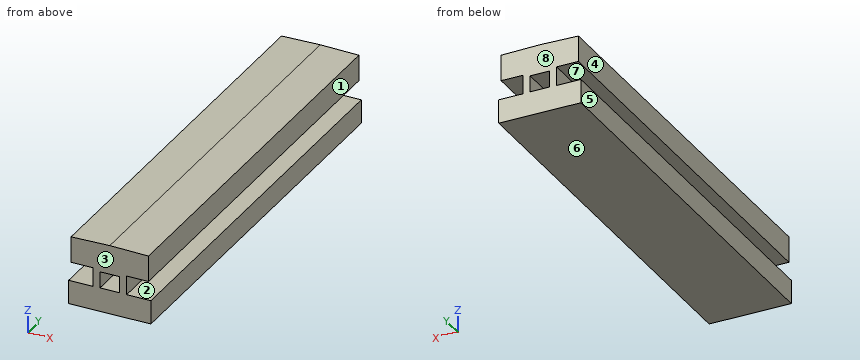
```python
from build123d import *

# Parameters (mm, degrees)
F1_DEPTH = 500
F2_W     = 23.519294
F2_H     = 19.81963
F3_DEPTH = 500


with BuildPart() as f1:
    # F0 (on Front) → F1 (new body)
    with BuildSketch(Plane.XZ):
        Polygon((-49.813338, -38.97861), (0, -38.97861), (49.813338, -38.97861), (49.813338, -10.174078), (20.480286, -10.174078), (20.480286, 12.816695), (46.90646, 12.816695), (46.90646, 44.263847), (0, 45.320891), (-46.90646, 44.263847), (-46.90646, 12.816695), (-20.480286, 12.816695), (-20.480286, -10.174078), (-49.813338, -10.174078), align=None)
    extrude(amount=F1_DEPTH)

    # F2 (on face) → F3 (cut)
    with BuildSketch(Plane.XZ.offset(500)):
        Rectangle(F2_W, F2_H)
    extrude(amount=-F3_DEPTH, mode=Mode.SUBTRACT)


solid = f1.part
```
Geometry check sheet. Reference: the model listing, model coordinates, mm. Face numbers are marked on the shaded views. A direction names the side the tool comes from. Round coordinates to 2 decimals unless told otherwise and drop trailing zeros. Write each loop counter-clockwise with the first axis right and the second up, starting at its lowest first coordinate (ties: lowest second). Pieces come first, ordered by that corner, then holes. Notation, with made-up numbers: (54, 34.25) -> (69, 34.25) arc R21 cw to (69, 58.25) -> close; hole circle Ø7 at (62, 28.25). An arc over 180 degrees is marked (long way). Put each result on its own line as item: value.
1) Thickness scan on probe 1 along X at (y, z) = (-355, 1); probe 2 along Z at (x, y) = (45, -41.5); probe 3 along X at (y, z) = (-142.5, 23). Record the ranges inside material, lowest first. Write a range as from..to.
Recorded:
probe 1: x = -20.48..-11.76, 11.76..20.48
probe 2: z = -38.98..-10.17, 12.82..44.31
probe 3: x = -46.91..46.91
2) Release check for a two-part mould opening along Z. For the marked faces 6, 7 and 8 record: pulls with the +Z half, pulls with the -Z half, needs draft (parallel to the pull), parting line crosses it, or undercut.
Recorded:
face 6: pulls with the -Z half
face 7: undercut
face 8: needs draft
3) Cross-section at A-A, the plane z = -2. Enter the section's corners in (x, y), plus the area to 3 significant figures.
Recorded:
outline: (-20.48, -500) -> (-11.76, -500) -> (-11.76, 0) -> (-20.48, 0) -> close; (11.76, -500) -> (20.48, -500) -> (20.48, 0) -> (11.76, 0) -> close
area: 8,720 mm2
4) Access from +Z, -Z, +X, -X, +Y, -Y to the whole of each face (thin tool, end or side, straight path). Record for the marked faces 1, 2, 3, 4 and 5.
Recorded:
face 1: +Z, +X, +Y, -Y
face 2: +X, +Y, -Y
face 3: +Z, -Z, +X, -X, -Y
face 4: +Z, -X, +Y, -Y
face 5: +Z, -Z, -X, +Y, -Y
5) Cross-section at B-B, the plane y = -334. Enter the section's corners in (x, z).
Recorded:
outline: (-49.81, -38.98) -> (49.81, -38.98) -> (49.81, -10.17) -> (20.48, -10.17) -> (20.48, 12.82) -> (46.91, 12.82) -> (46.91, 44.26) -> (0, 45.32) -> (-46.91, 44.26) -> (-46.91, 12.82) -> (-20.48, 12.82) -> (-20.48, -10.17) -> (-49.81, -10.17) -> close; hole (-11.76, -9.91) -> (11.76, -9.91) -> (11.76, 9.91) -> (-11.76, 9.91) -> close
6) Cross-section at C-C, the plane x = 26. Enter the section's corners in (y, z), plus the area to 3 significant figures.
Recorded:
outline: (-500, -38.98) -> (0, -38.98) -> (0, -10.17) -> (-500, -10.17) -> close; (-500, 12.82) -> (0, 12.82) -> (0, 44.73) -> (-500, 44.73) -> close
area: 30,400 mm2
7) Cross-section at D-D, the plane z = 36. Enter the section's corners in (x, y), plus the area to 3 significant figures.
Recorded:
outline: (-46.91, -500) -> (46.91, -500) -> (46.91, 0) -> (-46.91, 0) -> close
area: 46,900 mm2
8) Depth check by flat-ended pin: P1, Ø11.5, axis at y = -181.5, z = 0.5, coming from the -X side; P2, Ø1, axis at y = -171.5, z = 21.5, coming from the +X side; P3, Ø9, axis at x = -35, y = -136, coming from the +Z side; P4, Ø19, axis at x = 4, y = -276, coming from the +Z side. Enter the tip coordinate at first touch or a pass-through.
Recorded:
P1: stops at x = -20.48
P2: stops at x = 46.91
P3: stops at z = 44.63
P4: stops at z = 45.32
